Model file for the job. Use its own axes, mm. A direction names the side the tool comes from. Coordinates: 2 decimals unless noted, no trailing zeros. Order: outer loops, then holes, each group sorted by start corner. A loop starts at its lowest first (then second) coordinate and runs counter-clockwise, first axis right, second up. Notation, with made-up numbers: (55.5, 84) -> (62.5, 84) arc R17 ccw to (62.5, 89) -> close; hole circle Ø1 at (17, -34). An arc over 180 degrees is marked (long way). Return JSON: item names as keys, results as strings. Group by question number.
1) Cut at A-A (y = 12.5). Write the cut outline in (x, z), and give its area (3 significant figures).
2) Cut at D-D (x = 61.5). Write the cut outline in (y, z) (3 decimals).
3) Probe line 1 (X direction, y = -2.5, z = 61.5); line 2 (X direction, y = -6, z = 6.5). List the from-to ranges inside material, lowest first.
4) Flat gauge pins, fed straight in: pin 1 (22 mm diameter, centred on y = 5.5, z = 48.5, fed in from +X); pin 2 (3 mm diameter, centred on x = 26.5, z = 46.5, fed in from +Y); pin 3 (1.5 mm diameter, centred on x = 24, y = -7.5, fed in from -Z). Where does each tip first touch, or does it go through?
5) Which spindle directions (+Z, -Z, +X, -X, +Y, -Y) get a long thin tool onto all of the face, cutting with end or side? Do faces 1 (the cylindrical face through (-2.46, -8.43, 29.68)), 2 (the flat face through (59, -5, 0)), 3 (the flat face through (50, 0, -5)). Say none if no direction does.
6) Cut at B-B (y = 0). Write the cut outline in (x, z).
7) Cut at C-C (z = 65). Write the cut outline in (x, y).
from build123d import *

# Parameters (mm, degrees)
SWEEP_2_PROFILE_R = 10
SKETCH_11_R       = 22
EXTRUDE_4_DEPTH   = 5
SKETCH_16_R       = 22
EXTRUDE_7_DEPTH   = 5


with BuildPart() as part:
    # 扫描2: sweep along a path in 草图1
    with BuildLine(Plane(origin=(0, 0, 0), x_dir=(1, 0, 0), z_dir=(0, 1, 0))) as sweep_2_path:
        ThreePointArc((50, 0), (35.3553, -35.3553), (0, -50))
    # 扫描2 profile (on start of the path) → 扫描2 (sweep)
    with BuildSketch(Plane(origin=(50, 0, 0), x_dir=(0.9999999999964432, 0, 2.6671391793895655e-06), z_dir=(-2.6671391793895655e-06, 0, 0.9999999999964432))):
        Circle(SWEEP_2_PROFILE_R)
    sweep(path=sweep_2_path.line)

    # 草图11 → 凸台-拉伸4 (add)
    with BuildSketch(Plane.XY):
        with Locations((50, 0)):
            Circle(SKETCH_11_R)
    extrude(amount=-EXTRUDE_4_DEPTH)

    # 草图16 → 凸台-拉伸7 (add)
    with BuildSketch(Plane(origin=(0, 0, 0), x_dir=(0, 0, -1), z_dir=(1, 0, 0))):
        with Locations((-50, 0)):
            Circle(SKETCH_16_R)
    extrude(amount=-EXTRUDE_7_DEPTH)


solid = part.part
Answers below:
{
 "1": {"outline": "(-5, 31.9) -> (0, 31.9) -> (0, 68.1) -> (-5, 68.1) -> close; (31.9, -5) -> (68.1, -5) -> (68.1, 0) -> (31.9, 0) -> close", "area": "362 mm^2"},
 "2": {"outline": "(-18.755, -5) -> (18.755, -5) -> (18.755, 0) -> (-18.755, 0) -> close"},
 "3": {"line 1": "x = -5 to 0", "line 2": "x = 41.49 to 57.63"},
 "4": {"pin 1": "stops at x = 46.11", "pin 2": "stops at y = 9.79", "pin 3": "stops at z = 35.08"},
 "5": {"face 1": "-X", "face 2": "none", "face 3": "-Z, +X, -X, +Y, -Y"},
 "6": {"outline": "(-5, 28) -> (0, 28) -> (0, 40) arc R40 cw to (40, 0) -> (28, 0) -> (28, -5) -> (72, -5) -> (72, 0) -> (50, 0) -> (60, 0) arc R60 ccw to (0, 60) -> (0, 50) -> (0, 72) -> (-5, 72) -> close"},
 "7": {"outline": "(-5, -16.09) -> (0, -16.09) -> (0, 16.09) -> (-5, 16.09) -> close"}
}
